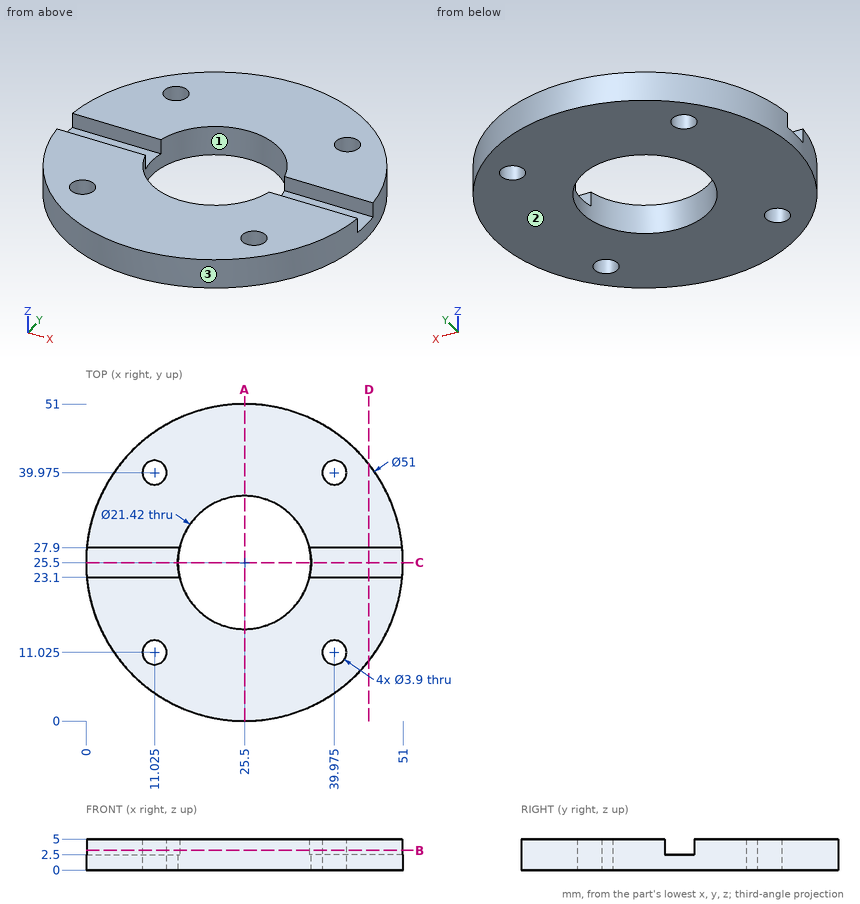
Can you work these out from the drawing? Everything is in mm from the part's minimum corner. Coordinates: 2 decimals unless noted, no trailing zeros. Write each loop counter-clockwise with the first axis right and the second up, starting at its lowest first coordinate (ties: lowest second). Pieces come first, ordered by that corner, then holes. Notation, with made-up numbers: (-8, -3.75) -> (3, -3.75) arc R25 cw to (3, 15.25) -> close; hole circle Ø3 at (-18.75, 77). An arc over 180 degrees is marked (long way). Write each question's results on one line, items separated by ' | '. Start each with the question number.
Item 1: If we section it at D-D, the plane x = 45.5: Write out the boundary of the cut face in (y, z).
Item 2: If we section it at A-A, the plane x = 25.5: Write out the boundary of the cut face in (y, z).
Item 3: If we section it at B-B, the plane z = 3.15: Write out the boundary of the cut face in (x, y) (3 decimals).
Item 4: Thinking about a two-plate mould opening in Y: for the marked faces 1, 2 and 3, which applies, released by +Y, released by -Y, zero draft, split by the parting line, or undercut?
Item 5: Please list where these lines run through material, in increasing order: probe 1 along X at (y, z) = (10, 1.85); probe 2 along X at (y, z) = (9.5, 1.2); probe 3 along Y at (x, z) = (39.5, 4.5).
Item 6: I'm going to push flat-ended pins straight in: P1, Ø1.4, axis at x = 40.5, y = 25, coming from the +Z side; P2, Ø1.2, axis at x = 5.5, z = 4, coming from the -Y side; P3, Ø3.5, axis at x = 11.025, y = 11.025, coming from the -Z side (3 decimals); P4, Ø3, axis at x = 44, z = 4, coming from the -Y side. Where does each tip first touch, or does it pass through?
Item 7: If we section it at C-C, the plane y = 25.5: Write out the boundary of the cut face in (x, z), and give its area (4 significant figures).
Answer block:
1) outline: (9.68, 0) -> (41.32, 0) -> (41.32, 5) -> (27.9, 5) -> (27.9, 2.5) -> (23.1, 2.5) -> (23.1, 5) -> (9.68, 5) -> close
2) outline: (0, 0) -> (14.79, 0) -> (14.79, 5) -> (0, 5) -> close; (36.21, 0) -> (51, 0) -> (51, 5) -> (36.21, 5) -> close
3) outline: (0.113, 23.1) arc R25.5 ccw to (50.887, 23.1) -> (35.938, 23.1) arc R10.71 cw to (15.062, 23.1) -> close; (0.113, 27.9) -> (15.062, 27.9) arc R10.71 cw to (35.938, 27.9) -> (50.887, 27.9) arc R25.5 ccw to start; hole circle Ø3.9 at (11.025, 11.025); hole circle Ø3.9 at (11.025, 39.975); hole circle Ø3.9 at (39.975, 11.025); hole circle Ø3.9 at (39.975, 39.975)
4) face 1: undercut | face 2: zero draft | face 3: split by the parting line
5) probe 1: 5.25 to 9.37, 12.68 to 38.32, 41.63 to 45.75 | probe 2: 5.64 to 9.81, 12.24 to 38.76, 41.19 to 45.36 | probe 3: 4.19 to 9.13, 12.92 to 23.1, 27.9 to 38.08, 41.87 to 46.81
6) P1: z = 2.5 | P2: y = 8.95 | P3: through | P4: y = 6.49
7) outline: (0, 0) -> (14.79, 0) -> (14.79, 2.5) -> (0, 2.5) -> close; (36.21, 0) -> (51, 0) -> (51, 2.5) -> (36.21, 2.5) -> close | area: 73.95 mm²
